Here's how the part is built. I have some questions about the finished solid (model axes, mm). A direction names the side the tool comes from. Give positions to 0.01 mm unless a question says otherwise; leave off trailing zeros. Write each loop counter-clockwise with the first axis right and the second up, starting at its lowest first coordinate (ties: lowest second). Pieces come first, ordered by that corner, then holes. Notation, with made-up numbers: (17, 87.5) -> (47, 87.5) arc R15 cw to (47, 107.5) -> close; hole circle Ø7 at (-22, 68). An arc over 180 degrees is marked (long way). Use CSV: the item, a comma, the result in double quotes. Start each with the question number.
(1) Which directions (+Z, -Z, +X, -X, +Y, -Y) give clear straight access to the entire face, cutting with the end or side of a thin tool? Please do faces 1 (the flat face through (-21.209, 0, -44)), 2 (the flat face through (0, -21.109, -24)), 3 (the cylindrical face through (17.732, -17.623, -23.786)), 4 (the cylindrical face through (-18.701, 18.776, -43.686)), 5 (the cylindrical face through (16.421, 16.345, -6.76)).
(2) I need wall thicknesses on L1, parallel to Y at x = 15.5, z = -4.7; L2, parallel to Y at x = -15.5, z = -6.8. Which ranges of each line are inside material? Lowest first, please. Write a range as [from, to].
(3) Suppose I cut it at C-C on x = 0. List the corners of the cut face in (y, z) for me.
(4) For pin 1 Ø2.5 at (x, y) = (-15, -16) entering from +Z; pin 2 Ø0.9 at (x, y) = (15.5, -16) entering from +Z; pin 3 Ø13.5 at (x, z) = (0.5, -16.5) entering from +Y, each with a flat end and sliding along its axis, tell me the tip position at first contact or that it passes through.
(5) Suppose I cut it at D-D on x = -6.5. List the corners of the cut face in (y, z) for me.
(6) If we mould it in two halves opening along Y, with no side actions, what happens to faces 6 (the cylindrical face through (18.701, -18.776, -4.436)), 7 (the cylindrical face through (2.38, -10.74, 0.99)), 8 (the cylindrical face through (-15.34, -14.26, -6.76))? For each: pulls with the +Y half, pulls with the -Y half, needs draft (parallel to the pull), parting line crosses it, or undercut.
(7) Suppose I cut it at B-B on y = 0. List the corners of the cut face in (x, z) for me.
(8) Suppose I cut it at A-A on z = -20.5. List the corners of the cut face in (x, y) for me.
from build123d import *

# Parameters (mm, degrees)
SKETCH1_R                       = 2.5
BOSS_EXTRUDE1_DEPTH             = 24
SKETCH2_R                       = 11
BOSS_EXTRUDE2_DEPTH             = 2
SKETCH3_W                       = 42.418
SKETCH3_H                       = 42.418
BOSS_EXTRUDE3_DEPTH             = 48
CUT_EXTRUDE1_DEPTH              = 73
M3X0_5_TAPPED_HOLE1_D           = 2.5
M3X0_5_TAPPED_HOLE1_DEPTH       = 7.5
M3X0_5_TAPPED_HOLE1_CBORE_D     = 3
M3X0_5_TAPPED_HOLE1_CBORE_DEPTH = 6
M3X0_5_TAPPED_HOLE1_TIP         = 0.751075774
CUT_EXTRUDE2_DEPTH              = 15
CUT_EXTRUDE3_DEPTH              = 15.25


with BuildPart() as part:
    # Sketch1 → Boss-Extrude1 (new body)
    with BuildSketch(Plane.XY):
        Circle(SKETCH1_R)
    extrude(amount=BOSS_EXTRUDE1_DEPTH)

    # Sketch2 → Boss-Extrude2 (add)
    with BuildSketch(Plane(origin=(0, 0, 0), x_dir=(-1, 0, 0), z_dir=(0, 0, -1))):
        Circle(SKETCH2_R)
    extrude(amount=-BOSS_EXTRUDE2_DEPTH)

    # Sketch3 → Boss-Extrude3 (add)
    with BuildSketch(Plane(origin=(0, 0, 0), x_dir=(-1, 0, 0), z_dir=(0, 0, -1))):
        Rectangle(SKETCH3_W, SKETCH3_H)
    extrude(amount=BOSS_EXTRUDE3_DEPTH)

    # Sketch4 → Cut-Extrude1 (cut, through all)
    with BuildSketch(Plane(origin=(0, 0, -48), x_dir=(-1, 0, 0), z_dir=(0, 0, -1))):
        with BuildLine():
            Line((-21.209, -15.887992919), (-21.209, -21.209))
            Line((-21.209, -21.209), (-15.887992919, -21.209))
            ThreePointArc((-15.887992919, -21.209), (-18.738329701, -18.738329701), (-21.209, -15.887992919))
        make_face()
        with BuildLine():
            Line((15.887992919, -21.209), (21.209, -21.209))
            Line((21.209, -21.209), (21.209, -15.887992919))
            ThreePointArc((21.209, -15.887992919), (18.738329701, -18.738329701), (15.887992919, -21.209))
        make_face()
        with BuildLine():
            Line((21.209, 15.887992919), (21.209, 21.209))
            Line((21.209, 21.209), (15.887992919, 21.209))
            ThreePointArc((15.887992919, 21.209), (18.738329701, 18.738329701), (21.209, 15.887992919))
        make_face()
        with BuildLine():
            Line((-15.887992919, 21.209), (-21.209, 21.209))
            Line((-21.209, 21.209), (-21.209, 15.887992919))
            ThreePointArc((-21.209, 15.887992919), (-18.738329701, 18.738329701), (-15.887992919, 21.209))
        make_face()
    extrude(amount=-CUT_EXTRUDE1_DEPTH, mode=Mode.SUBTRACT)

    # M3x0.5 Tapped Hole1
    with Locations(Plane.XY):
        with Locations((-15.5, 15.5), (-15.5, -15.5), (15.5, -15.5), (15.5, 15.5)):
            CounterBoreHole(M3X0_5_TAPPED_HOLE1_D / 2, M3X0_5_TAPPED_HOLE1_CBORE_D / 2, M3X0_5_TAPPED_HOLE1_CBORE_DEPTH, depth=M3X0_5_TAPPED_HOLE1_DEPTH)
            with Locations((0, 0, -(M3X0_5_TAPPED_HOLE1_DEPTH + M3X0_5_TAPPED_HOLE1_TIP / 2))):  # 118° drill point
                Cone(0, M3X0_5_TAPPED_HOLE1_D / 2, M3X0_5_TAPPED_HOLE1_TIP, mode=Mode.SUBTRACT)

    # Sketch7 → Cut-Extrude2 (cut)
    with BuildSketch(Plane.XY.offset(24)):
        with BuildLine():
            Line((-1.5, 2), (1.5, 2))
            ThreePointArc((1.5, 2), (0, 2.5), (-1.5, 2))
        make_face()
    extrude(amount=-CUT_EXTRUDE2_DEPTH, mode=Mode.SUBTRACT)

    # Sketch8 → Cut-Extrude3 (cut, symmetric)
    with BuildSketch(Plane.XY.offset(-24)):
        with BuildLine():
            Line((15.887992919, 21.209), (-15.887992919, 21.209))
            ThreePointArc((-15.887992919, 21.209), (-18.738329701, 18.738329701), (-21.209, 15.887992919))
            Line((-21.209, 15.887992919), (-21.209, -15.887992919))
            ThreePointArc((-21.209, -15.887992919), (-18.738329701, -18.738329701), (-15.887992919, -21.209))
            Line((-15.887992919, -21.209), (15.887992919, -21.209))
            ThreePointArc((15.887992919, -21.209), (18.738329701, -18.738329701), (21.209, -15.887992919))
            Line((21.209, -15.887992919), (21.209, 15.887992919))
            ThreePointArc((21.209, 15.887992919), (18.738329701, 18.738329701), (15.887992919, 21.209))
        make_face()
        with BuildLine():
            Line((-13.394406258, 21.109), (13.394406258, 21.109))
            ThreePointArc((13.394406258, 21.109), (17.67766953, 17.67766953), (21.109, 13.394406258))
            Line((21.109, 13.394406258), (21.109, -13.394406258))
            ThreePointArc((21.109, -13.394406258), (17.67766953, -17.67766953), (13.394406258, -21.109))
            Line((13.394406258, -21.109), (-13.394406258, -21.109))
            ThreePointArc((-13.394406258, -21.109), (-17.67766953, -17.67766953), (-21.109, -13.394406258))
            Line((-21.109, -13.394406258), (-21.109, 13.394406258))
            ThreePointArc((-21.109, 13.394406258), (-17.67766953, 17.67766953), (-13.394406258, 21.109))
        make_face(mode=Mode.SUBTRACT)
    extrude(amount=CUT_EXTRUDE3_DEPTH, both=True, mode=Mode.SUBTRACT)


solid = part.part
Geometry says:
1,face 1,"+Z, -Z, -X, +Y, -Y"
1,face 2,"+X, -X, -Y"
1,face 3,"+X, -Y"
1,face 4,"+Z, -Z, -X, +Y"
1,face 5,"+Z"
2,L1,"[-21.21, -17], [-14, 14], [17, 21.21]"
2,L2,"[-21.21, -16.75], [-14.25, 14.25], [16.75, 21.21]"
3,outline,"(-21.21, -48) -> (21.21, -48) -> (21.21, -39.25) -> (21.11, -39.25) -> (21.11, -8.75) -> (21.21, -8.75) -> (21.21, 0) -> (11, 0) -> (11, 2) -> (2.5, 2) -> (2.5, 9) -> (2, 9) -> (2, 24) -> (-2.5, 24) -> (-2.5, 2) -> (-11, 2) -> (-11, 0) -> (-21.21, 0) -> (-21.21, -8.75) -> (-21.11, -8.75) -> (-21.11, -39.25) -> (-21.21, -39.25) -> close"
4,pin 1,"z = 0"
4,pin 2,"z = -7.68"
4,pin 3,"y = 21.11"
5,outline,"(-21.21, -48) -> (21.21, -48) -> (21.21, -39.25) -> (21.11, -39.25) -> (21.11, -8.75) -> (21.21, -8.75) -> (21.21, 0) -> (8.87, 0) -> (8.87, 2) -> (-8.87, 2) -> (-8.87, 0) -> (-21.21, 0) -> (-21.21, -8.75) -> (-21.11, -8.75) -> (-21.11, -39.25) -> (-21.21, -39.25) -> close"
6,face 6,"pulls with the -Y half"
6,face 7,"parting line crosses it"
6,face 8,"undercut"
7,outline,"(-21.21, -48) -> (21.21, -48) -> (21.21, -39.25) -> (21.11, -39.25) -> (21.11, -8.75) -> (21.21, -8.75) -> (21.21, 0) -> (11, 0) -> (11, 2) -> (2.5, 2) -> (2.5, 24) -> (-2.5, 24) -> (-2.5, 2) -> (-11, 2) -> (-11, 0) -> (-21.21, 0) -> (-21.21, -8.75) -> (-21.11, -8.75) -> (-21.11, -39.25) -> (-21.21, -39.25) -> close"
8,outline,"(-21.11, -13.39) arc R25 ccw to (-13.39, -21.11) -> (13.39, -21.11) arc R25 ccw to (21.11, -13.39) -> (21.11, 13.39) arc R25 ccw to (13.39, 21.11) -> (-13.39, 21.11) arc R25 ccw to (-21.11, 13.39) -> close"
